The drawing under review shows one solid part. Ordinate dimensions are in mm from its lowest x, y, z. A direction names the side the tool comes from. Give positions to 0.01 mm unless a question says otherwise; leave off trailing zeros. Order: outer loops, then holes, each group sorted by start corner. A loop starts at its lowest first (then second) coordinate and runs counter-clockwise, first axis right, second up. Notation, with made-up numbers: (-38.5, -24.75) - (19.5, -24.75) arc R14 ccw to (19.5, -11.75) - close; hole circle Ø1 at (49, 8). An arc over 180 degrees is marked (long way). Answer as a JSON object with one key per item and string values. Group by question number.
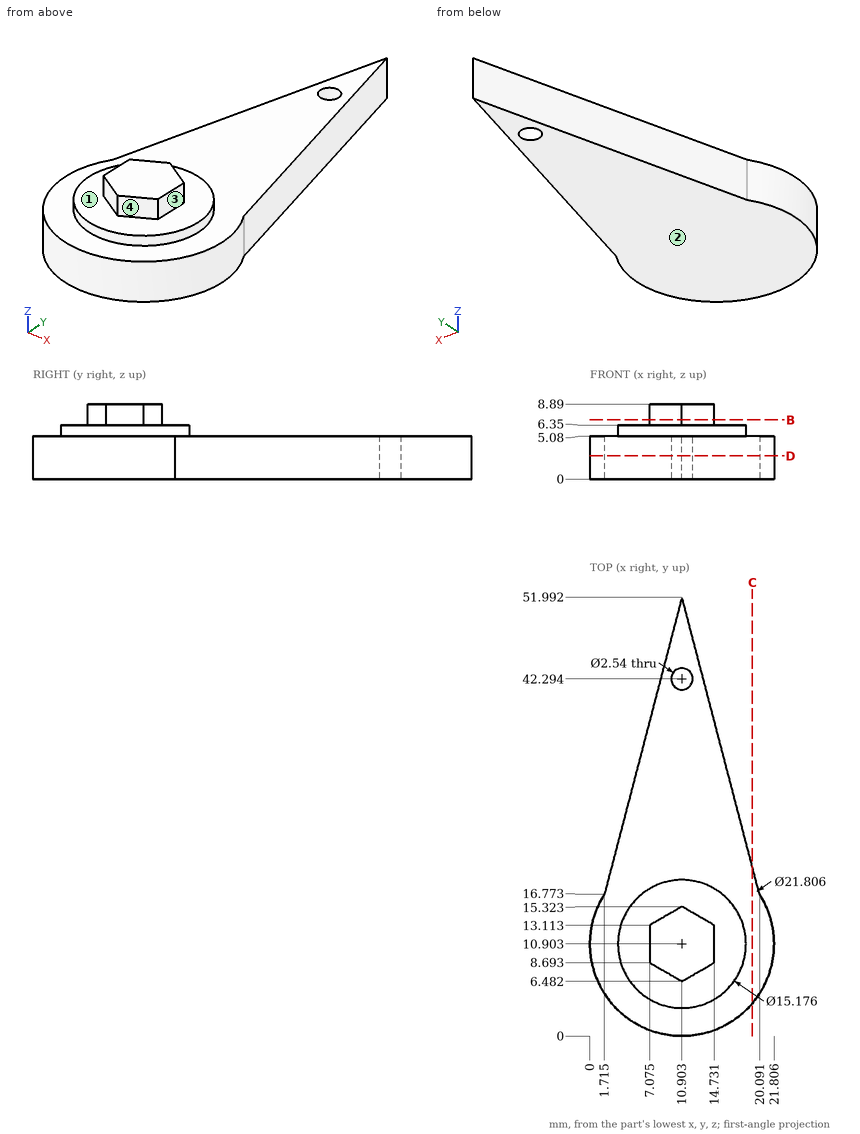
1) For the marked faces 1, 2, 3 and 4, list the 3-axis set-ups (+Z, -Z, +X, -X, +Y, -Y) from which the entire face can be reached by the end or side of a thin tool; tool diameter is ignored.
2) For line 1 (Z direction, x = 9, y = 26); line 2 (Z direction, x = 13.75, y = 15); line 3 (X direction, y = 11, z = 2.5) (1 decimal), list the stretches that pass through material, from the lowest coordinate up.
3) For pin 1 (3 mm diameter, centred on x = 17.5, y = 23, fed in from +Z); pin 2 (1.5 mm diameter, centred on x = 5.5, y = 19.5, fed in from -Z); pin 3 (3 mm diameter, centred on y = 10, z = 7, fed in from +X); pin 4 (0.8 mm diameter, centred on y = 12, z = 7, fed in from -X) (1 decimal), all flat-tipped, find the tip position at first contact; note any pin that passes through.
4) Consider section D-D (z = 2.75). Give the boundary of the cut face in (x, y) (1 decimal).
5) Consider section C-C (x = 19.25). Give the boundary of the cut face in (y, z) (1 decimal).
6) Consider section B-B (z = 7). Give the boundary of the cut face in (x, y) (1 decimal).
Result set:
{
 "1": {"face 1": "+Z", "face 2": "-Z, +X, -X, +Y, -Y", "face 3": "+Z, +X, +Y, -Y", "face 4": "+Z, +X, -Y"},
 "2": {"line 1": "z = 0 to 5.08", "line 2": "z = 0 to 6.35", "line 3": "x = 0 to 21.8"},
 "3": {"pin 1": "stops at z = 5.08", "pin 2": "stops at z = 0", "pin 3": "stops at x = 18.49", "pin 4": "stops at x = 7.1"},
 "4": {"outline": "(1.7, 16.8) arc R10.9 ccw (long way) to (20.1, 16.8) - (10.9, 52) - close; hole circle Ø2.5 at (10.9, 42.3)"},
 "5": {"outline": "(3.9, 0) - (20, 0) - (20, 5.1) - (3.9, 5.1) - close"},
 "6": {"outline": "(7.1, 8.7) - (10.9, 6.5) - (14.7, 8.7) - (14.7, 13.1) - (10.9, 15.3) - (7.1, 13.1) - close"}
}
